```python
from build123d import *

# Parameters (mm, degrees)
AUFSATZ_LINEAR_AUSTRAGEN1_DEPTH                      = 20
STIRNSENKUNG_F_R_M3_ZYLINDERSCHRAUBE_MIT_D           = 3.6
STIRNSENKUNG_F_R_M3_ZYLINDERSCHRAUBE_MIT_DEPTH       = 17
STIRNSENKUNG_F_R_M3_ZYLINDERSCHRAUBE_MIT_CBORE_D     = 6.5
STIRNSENKUNG_F_R_M3_ZYLINDERSCHRAUBE_MIT_CBORE_DEPTH = 3.4


with BuildPart() as part:
    # Skizze1 → Aufsatz-Linear austragen1 (new body)
    with BuildSketch(Plane.XY):
        Polygon((5, 0), (20, 0), (25, 5), (25, 38), (30, 43), (140, 43), (145, 38), (145, 5), (150, 0), (165, 0), (170, -5), (170, -17), (140, -17), (135, -12), (135, 28), (130, 33), (40, 33), (35, 28), (35, -12), (30, -17), (0, -17), (0, -5), align=None)
    extrude(amount=AUFSATZ_LINEAR_AUSTRAGEN1_DEPTH)

    # Stirnsenkung für M3 Zylinderschraube mit Innensechskant2
    with Locations(Plane(origin=(0, 0, 0), x_dir=(1, 0, 0), z_dir=(0, 1, 0))):
        with Locations((157.5, -10), (12.5, -10)):
            CounterBoreHole(STIRNSENKUNG_F_R_M3_ZYLINDERSCHRAUBE_MIT_D / 2, STIRNSENKUNG_F_R_M3_ZYLINDERSCHRAUBE_MIT_CBORE_D / 2, STIRNSENKUNG_F_R_M3_ZYLINDERSCHRAUBE_MIT_CBORE_DEPTH, depth=STIRNSENKUNG_F_R_M3_ZYLINDERSCHRAUBE_MIT_DEPTH)


solid = part.part
```
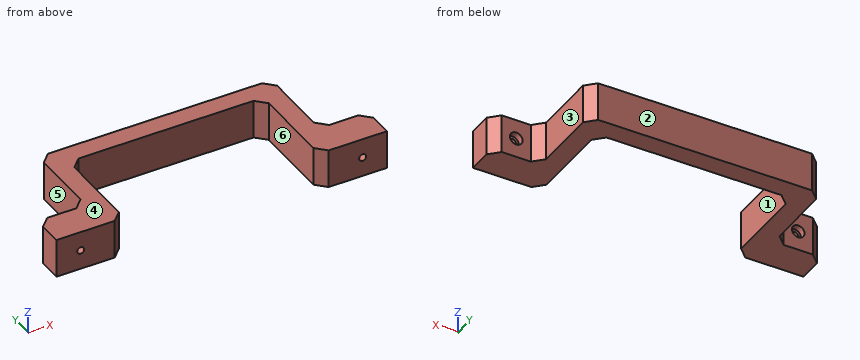
Geometry check sheet. Reference: the model listing, model coordinates, mm. Face numbers are marked on the shaded views. A direction names the side the tool comes from. Give positions to 0.01 mm unless a question says otherwise; leave off trailing zeros. Loops run counter-clockwise (first coordinate to the right, second up) from the corner with the lowest first, then second, coordinate; pieces in that order, holes last. Notation, with made-up numbers: M 65.25,11 L 108.25,11 A17 ccw 108.25,38 Z; hole C 20,-5.75 d7. An arc over 180 degrees is marked long. Answer as CSV lines item,"result".
Item 1: Cross-section at C-C on y = 29.5. Record the cut outline in (x, z), and give its area (3 significant figures).
Values:
outline,"M 25,0 L 36.5,0 L 36.5,20 L 25,20 Z; M 133.5,0 L 145,0 L 145,20 L 133.5,20 Z"
area,"460 mm²"
Item 2: Depth check by flat-ended pin: P1, Ø2, axis at x = 13.5, z = 11.5, coming from the +Y side; P2, Ø6, axis at y = 7.5, z = 6.5, coming from the -X side; P3, Ø6, axis at y = 26, z = 6.5, coming from the +X side. Enter the tip coordinate at first touch or a pass-through.
Values:
P1,"stops at y = -3.4"
P2,"stops at x = 24.5"
P3,"stops at x = 145"
Item 3: Release check for a two-part mould opening along X. For the marked faces 1, 2 and 3 record: pulls with the +X half, pulls with the -X half, needs draft (parallel to the pull), parting line crosses it, or undercut.
Values:
face 1,"undercut"
face 2,"needs draft"
face 3,"pulls with the +X half"
Item 4: Cross-section at B-B on x = 12.5. Record the cut outline in (y, z), and give its area (3 significant figures).
Values:
outline,"M -17,0 L 0,0 L 0,6.75 L -3.4,6.75 L -3.4,8.2 L -17,8.2 Z; M -17,11.8 L -3.4,11.8 L -3.4,13.25 L 0,13.25 L 0,20 L -17,20 Z"
area,"269 mm²"
Item 5: Access from +Z, -Z, +X, -X, +Y, -Y to the whole of each face (thin tool, end or side, straight path). Record for the marked faces 4, 5 and 6.
Values:
face 4,"+Z, +X, -X, +Y, -Y"
face 5,"+Z, -Z, -X, +Y"
face 6,"+Z, -Z, -Y"
Item 6: Cross-section at D-D on z = 5. Record the cut outline in (x, y).
Values:
outline,"M 0,-17 L 30,-17 L 35,-12 L 35,28 L 40,33 L 130,33 L 135,28 L 135,-12 L 140,-17 L 170,-17 L 170,-5 L 165,0 L 150,0 L 145,5 L 145,38 L 140,43 L 30,43 L 25,38 L 25,5 L 20,0 L 5,0 L 0,-5 Z"
Item 7: Cross-section at A-A on y = -9. Record the cut outline in (x, z), and give its area (3 significant figures).
Values:
outline,"M 0,0 L 35,0 L 35,20 L 0,20 Z; M 135,0 L 170,0 L 170,20 L 135,20 Z; hole C 12.5,10 d3.6; hole C 157.5,10 d3.6"
area,"1,380 mm²"
Item 8: Material ranges on line 1 (Z direction, x = 157.5, y = -7.25); line 2 (X direction, y = -8, z = 10); line 3 (X direction, y = 12.5, z = 16), recorded low to high.
Values:
line 1,"z = 0 to 8.2, 11.8 to 20"
line 2,"x = 0 to 10.7, 14.3 to 35, 135 to 155.7, 159.3 to 170"
line 3,"x = 25 to 35, 135 to 145"
